from build123d import *

# Parameters (mm, degrees)
IZIM1_W                     = 20
IZIM1_H                     = 18.5
Y_KSEKLIK_EKSTR_ZYON1_DEPTH = 17
IZIM2_W                     = 20
IZIM2_H                     = 2
Y_KSEKLIK_EKSTR_ZYON2_DEPTH = 2
IZIM3_W                     = 20
IZIM3_H                     = 2
Y_KSEKLIK_EKSTR_ZYON3_DEPTH = 2
IZIM4_W                     = 20
IZIM4_H                     = 35
Y_KSEKLIK_EKSTR_ZYON4_DEPTH = 23
PAH1_SIZE                   = 7
PAH1_SIZE_2                 = 10
PAH2_SIZE                   = 7
PAH2_SIZE_2                 = 10
IZIM5_W                     = 5.25
IZIM5_H                     = 26.25
KES_EKSTR_ZYON2_DEPTH       = 14.75
IZIM6_W                     = 2
IZIM6_H                     = 17.25
KES_EKSTR_ZYON3_DEPTH       = 14.75


with BuildPart() as part:
    # Çizim1 → Yükseklik-Ekstrüzyon1 (new body)
    with BuildSketch(Plane.XY):
        Rectangle(IZIM1_W, IZIM1_H)
    extrude(amount=Y_KSEKLIK_EKSTR_ZYON1_DEPTH)

    # Çizim2 → Yükseklik-Ekstrüzyon2 (add)
    with BuildSketch(Plane.XZ.offset(9.25)):
        with Locations((0, 1)):
            Rectangle(IZIM2_W, IZIM2_H)
    extrude(amount=Y_KSEKLIK_EKSTR_ZYON2_DEPTH)

    # Çizim3 → Yükseklik-Ekstrüzyon3 (add)
    with BuildSketch(Plane(origin=(0, 9.25, 0), x_dir=(1, 0, 0), z_dir=(0, 1, 0))):
        with Locations((0, -1)):
            Rectangle(IZIM3_W, IZIM3_H)
    extrude(amount=Y_KSEKLIK_EKSTR_ZYON3_DEPTH)

    # Çizim4 → Yükseklik-Ekstrüzyon4 (add)
    with BuildSketch(Plane.XY.offset(17)):
        Rectangle(IZIM4_W, IZIM4_H)
    extrude(amount=Y_KSEKLIK_EKSTR_ZYON4_DEPTH)

    # Pah1
    # the kernel refuses this chamfer: 10, 7 mm, written as the material it takes off along each edge
    with BuildSketch(Plane(origin=(-35.825599626, 17.5, 17), x_dir=(0, 0.045281396304095924, 0.9989742715149131), z_dir=(1, 0, 0))) as pah1_piece_1_section:
        Polygon((PAH1_SIZE * 0.998974271515, PAH1_SIZE * 0.0452813963041), (-PAH1_SIZE_2 * 0.0452813963041, PAH1_SIZE_2 * 0.998974271515), (0, 0), align=None)
    pah1_piece_1 = extrude(amount=71.651199251, mode=Mode.PRIVATE)
    pah1_piece_1 = split(pah1_piece_1, bisect_by=Plane(origin=(0, 9.25, 19.372622849), z_dir=(0, 1, 0)), keep=Keep.TOP, mode=Mode.PRIVATE)
    add(pah1_piece_1, mode=Mode.SUBTRACT)

    # Pah2
    # the kernel refuses this chamfer: 10, 7 mm, written as the material it takes off along each edge
    with BuildSketch(Plane(origin=(35.825599626, -17.5, 17), x_dir=(0, -0.045281396304095924, 0.9989742715149131), z_dir=(-1, 0, 0))) as pah2_piece_1_section:
        Polygon((PAH2_SIZE * 0.998974271515, PAH2_SIZE * 0.0452813963041), (-PAH2_SIZE_2 * 0.0452813963041, PAH2_SIZE_2 * 0.998974271515), (0, 0), align=None)
    pah2_piece_1 = extrude(amount=71.651199251, mode=Mode.PRIVATE)
    pah2_piece_1 = split(pah2_piece_1, bisect_by=Plane(origin=(0, -9.25, 19.372622849), z_dir=(0, -1, 0)), keep=Keep.TOP, mode=Mode.PRIVATE)
    add(pah2_piece_1, mode=Mode.SUBTRACT)

    # Çizim5 → Kes-Ekstrüzyon2 (cut)
    with BuildSketch(Plane.XY.offset(40)):
        with Locations((5.375, 0)):
            Rectangle(IZIM5_W, IZIM5_H)
    extrude(amount=-KES_EKSTR_ZYON2_DEPTH, mode=Mode.SUBTRACT)

    # Çizim6 → Kes-Ekstrüzyon3 (cut)
    with BuildSketch(Plane.XY.offset(40)):
        with Locations((9, 0)):
            Rectangle(IZIM6_W, IZIM6_H)
    extrude(amount=-KES_EKSTR_ZYON3_DEPTH, mode=Mode.SUBTRACT)


solid = part.part
Read the model definition and answer for the solid it produces. Units are mm, in the model's axes. A direction names the side the tool comes from. Coordinates: 2 decimals unless noted, no trailing zeros. Order: outer loops, then holes, each group sorted by start corner. A loop starts at its lowest first (then second) coordinate and runs counter-clockwise, first axis right, second up. Notation, with made-up numbers: (-38, -12.75) - (20, -12.75) arc R28 ccw to (20, 15.25) - close; hole circle Ø1 at (-39.5, 68). An arc over 180 degrees is marked (long way). Use one line per item in the form item = value.
(1) Section B-B, the plane z = 28.5 is taken. Give the vertices of the cut face in (x, y) (3 decimals), then the cut area to 3 significant figures.
Computed values:
outline = (-10, -17.5) - (10, -17.5) - (10, -8.625) - (8, -8.625) - (8, -13.125) - (2.75, -13.125) - (2.75, 13.125) - (8, 13.125) - (8, 8.625) - (10, 8.625) - (10, 17.5) - (-10, 17.5) - close
area = 528 mm²
(2) Given pin 1 Ø4 at (x, z) = (5, 17.5) entering from -Y; pin 2 Ø8 at (x, z) = (-2.5, 8) entering from +Y; pin 3 Ø2 at (x, y) = (7.5, 5.5) entering from +Z, each flat-ended and moving along its own axis, determine where each tip first touches the part or whether it passes through.
Computed values:
pin_1 = -11.07
pin_2 = 9.25
pin_3 = 25.25
(3) Which of the six approach directions +Z, -Z, +X, -X, +Y, -Y give full straight-line access (tool end or side, diameter ignored) to faces 1 (the face through (5, 13.125, 33)), 2 (the face through (0, 9.25, 10)), 3 (the face through (0.14, -13.43, 21.15)), 4 (the face through (9, -8.625, 33))?
Computed values:
face_1 = +Z
face_2 = +X, -X, +Y
face_3 = +X, -X, -Y
face_4 = +Z, +X
(4) Section D-D, the plane x = 4.75 is taken. Give the vertices of the cut face in (y, z) (3 decimals).
Computed values:
outline = (-17.5, 24) - (-9.25, 18.225) - (-9.25, 2) - (-11.25, 2) - (-11.25, 0) - (11.25, 0) - (11.25, 2) - (9.25, 2) - (9.25, 18.225) - (17.5, 24) - (17.5, 40) - (13.125, 40) - (13.125, 25.25) - (-13.125, 25.25) - (-13.125, 40) - (-17.5, 40) - close
(5) For a pull along X with two mould halves and no side action, classify faces 5 (the face through (0, 11.25, 1)), 6 (the face through (10, 0, 20)), 7 (the face through (8, -11, 33)) as pulls with the +X half, pulls with the -X half, needs draft (parallel to the pull), parting line crosses it, or undercut.
Computed values:
face_5 = needs draft
face_6 = pulls with the +X half
face_7 = undercut
(6) Straight lines are drawn through the part: L1, parallel to X at y = 9, z = 26; L2, parallel to Y at x = 5.5, z = 6.5; L3, parallel to X at y = 0, z = 38.5. For each, find the intervals that lie inside material, in ascending order.
Computed values:
L1 = -10 to 2.75, 8 to 10
L2 = -9.25 to 9.25
L3 = -10 to 2.75
(7) Section C-C, the plane y = 6.5 is taken. Give the vertices of the cut face in (x, z), then the cut area to 3 significant figures.
Computed values:
outline = (-10, 0) - (10, 0) - (10, 25.25) - (2.75, 25.25) - (2.75, 40) - (-10, 40) - close
area = 693 mm²
(8) Section A-A, the plane x = -0.5 is taken. Give the vertices of the cut face in (y, z) (3 decimals).
Computed values:
outline = (-17.5, 24) - (-9.25, 18.225) - (-9.25, 2) - (-11.25, 2) - (-11.25, 0) - (11.25, 0) - (11.25, 2) - (9.25, 2) - (9.25, 18.225) - (17.5, 24) - (17.5, 40) - (-17.5, 40) - close
